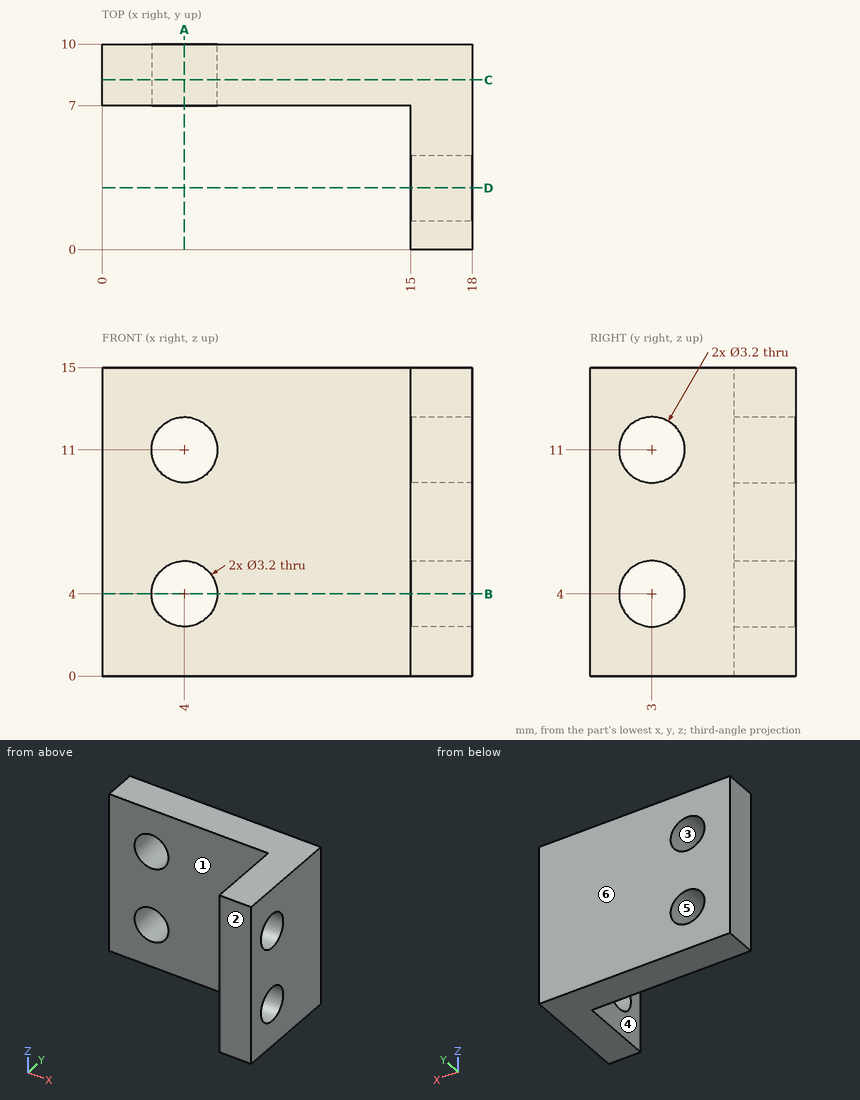
Can you work these out from the drawing? Everything is in mm from the part's minimum corner. A direction names the side the tool comes from. Give positions to 0.01 mm unless a question says otherwise; leave off trailing zeros. Order: outer loops, then holes, each group sorted by start corner. A loop starts at its lowest first (then second) coordinate and runs counter-clockwise, first axis right, second up. Notation, with made-up numbers: M 64,-7.75 L 95,-7.75 A15 cw 95,-2.75 Z; hole C 22.25,-13.5 d1. An arc over 180 degrees is marked long. One line per item, written item: value.
Item 1: For pin 1 (5 mm diameter, centred on y = 3.5, z = 5, fed in from +X); pin 2 (4 mm diameter, centred on y = 3, z = 11, fed in from -X); pin 3 (1 mm diameter, centred on x = 9.5, z = 9.5, fed in from -Y), each with a flat end and sliding along its axis, tell me the tip position at first contact or that it passes through.
Verdict:
pin 1: x = 18
pin 2: x = 15
pin 3: y = 7
Item 2: If we section it at C-C on y = 8.25: Write out the boundary of the cut face in (x, z).
Verdict:
outline: M 0,0 L 18,0 L 18,15 L 0,15 Z; hole C 4,4 d3.2; hole C 4,11 d3.2
Item 3: If we section it at D-D on y = 3: Write out the boundary of the cut face in (x, z).
Verdict:
outline: M 15,0 L 18,0 L 18,2.4 L 15,2.4 Z; M 15,5.6 L 18,5.6 L 18,9.4 L 15,9.4 Z; M 15,12.6 L 18,12.6 L 18,15 L 15,15 Z
Item 4: For the marked faces 1 and 2, which set-ups out of +Z, -Z, +X, -X, +Y, -Y let a thin tool reach every point of the face, with its end or its side?
Verdict:
face 1: +Z, -Z, -X, -Y
face 2: +Z, -Z, +X, -X, -Y
Item 5: Please list where these lines run through material, in increasing order: line 1 (Y direction, x = 15.85, z = 11); line 2 (Z direction, x = 4, y = 8); line 3 (Y direction, x = 9.25, z = 11.5).
Verdict:
line 1: 0 to 1.4, 4.6 to 10
line 2: 0 to 2.4, 5.6 to 9.4, 12.6 to 15
line 3: 7 to 10
Item 6: If we mould it in two halves opening along X, with no side actions, what happens to the marked faces 3, 4, 5 and 6? For each: pulls with the +X half, pulls with the -X half, needs draft (parallel to the pull), parting line crosses it, or undercut.
Verdict:
face 3: undercut
face 4: pulls with the -X half
face 5: undercut
face 6: needs draft
Item 7: If we section it at A-A on x = 4: Write out the boundary of the cut face in (y, z).
Verdict:
outline: M 7,0 L 10,0 L 10,2.4 L 7,2.4 Z; M 7,5.6 L 10,5.6 L 10,9.4 L 7,9.4 Z; M 7,12.6 L 10,12.6 L 10,15 L 7,15 Z
Item 8: If we section it at B-B on z = 4: Write out the boundary of the cut face in (x, y), and give its area (3 significant figures).
Verdict:
outline: M 0,7 L 2.4,7 L 2.4,10 L 0,10 Z; M 5.6,7 L 15,7 L 15,4.6 L 18,4.6 L 18,10 L 5.6,10 Z; M 15,0 L 18,0 L 18,1.4 L 15,1.4 Z
area: 55.8 mm2
